Geometry check sheet. Reference: the model listing, model coordinates, mm. A direction names the side the tool comes from. Round coordinates to 2 decimals unless told otherwise and drop trailing zeros. Write each loop counter-clockwise with the first axis right and the second up, starting at its lowest first coordinate (ties: lowest second). Pieces come first, ordered by that corner, then holes. Notation, with made-up numbers: (41.25, 56) - (47.25, 56) arc R18 ccw to (47.25, 71) - close; hole circle Ø5 at (-28, 55.5). An arc over 180 degrees is marked (long way). Return JSON: item names as keys, results as strings.
Autodesk Inventor part; units mm, degrees
ref_plane "Arbeitsebene1" through (0, 0, 7.5) normal (0, 0, 1) x (1, 0, 0)
ref_plane "YZ Plane" through (0, 0, 0) normal (1, 0, 0) x (0, 1, 0)
ref_plane "XZ Plane" through (0, 0, 0) normal (0, 1, 0) x (-1, 0, 0)
sketch "Skizze1" plane through (0, 0, 0) normal (0, 0, 1) x (1, 0, 0)
  line L0 (6.45, 0) -> (15, 0)
  line L1 (15, 0) -> (15, 15)
  line L2 (15, 15) -> (0, 15)
  line L3 (0, 15) -> (0, 3.0582)
  arc A0 (6.45, 0) -> (0, 3.0582) centre (2.5, 0) ccw
  line L4 (-3, 0) -> (18, 0)
  line L5 (0, -3) -> (0, 18)
  point P0 (0, 0)
  dimension "d0" = 15
  dimension "d1" = 15
  dimension "d2" = 7.9
  dimension "d3" = 2.5
extrude "Extrusion1" add sketch "Skizze1" along normal mid plane 17.5 contours A0 L3 L2 L1 L0
ref_plane "Arbeitsebene1" through (0, 0, 7.5) normal (0, 0, 1) x (1, 0, 0)
sketch "Skizze2" plane through (0, 0, 7.5) normal (0, 0, 1) x (1, 0, 0)
  circle A0 centre (2.5, 0) radius 3.95
  arc A1 (6.45, 0) -> (0, 3.0582) centre (2.5, 0) ccw
  circle A2 centre (2.5, 0) radius 3.45
  line L0 (0, 3.0582) -> (0, 2.3775)
  line L1 (15, 0) -> (6.45, 0)
  line L2 (6.45, 0) -> (5.95, 0)
  point P0 (0, 0)
  point P1 (0, 3.0582)
  dimension "d7" = 7.9
  dimension "d8" = 6.9
extrude "Extrusion2" add sketch "Skizze2" against normal up to surface (16.25 mm away) contours L2 A2 L0 A0 picked at (6.25, 0.2945)
sketch "Skizze4" plane through (15, 0, 8.75) normal (1, 0, 0) x (0, 0, -1)
  line L0 (17.5, 3) -> (0, 3)
  line L1 (0, 3) -> (0, 0)
  line L2 (0, 0) -> (17.5, 0)
  line L3 (17.5, 0) -> (17.5, 3)
  line L4 (17.5, 15) -> (17.5, 0)
  line L5 (0, 0) -> (0, 15)
  line L6 (17.5, 0) -> (0, 0)
  point P0 (8.75, 0)
  dimension "d11" = 3
extrude "Extrusion3" add sketch "Skizze4" along normal blind 13
fillet "Rundung1" radius 4 1 edges at (15, 3, 0)
sketch "Skizze5" plane through (28, 3, 8.75) normal (0, 1, 0) x (1, 0, 0)
  line L0 (-9, 0) -> (0, 0)
  line L1 (0, 17.5) -> (0, 0)
  point P0 (-28, 8.75)
  point P1 (-6.5, 10)
  dimension "d15" = 10
  dimension "d16" = 6.5
hole "Bohrung1" at (21.5, 3, -1.25) direction (0, -1, 0) diameter 4.1 end through all
sketch "Skizze6" plane through (5.95, 0, -8.75) normal (0, -1, 0) x (1, 0, 0)
  line L0 (0, 0) -> (22.05, 0)
  line L1 (-11.55, 8.75) -> (27.65, 8.75)
  line L2 (0, 16.25) -> (0, 0)
  point P0 (-5.95, 8.75)
  point P1 (6, 3)
  point P2 (6, 8.75)
  dimension "d24" = 3
  dimension "d25" = 6
hole "Bohrung2" at (11.95, 0, -5.75) at (11.95, 0, 0) direction (0, 1, 0) diameter 4 depth 8 tip angle 118
sketch "Skizze7" plane through (0, 0, -8.75) normal (0, 0, -1) x (-1, 0, 0)
  circle A0 centre (-2.5, 0) radius 6
  arc A1 (0, 2.3775) -> (-5.95, 0) centre (-2.5, 0) ccw
  line L0 (-5.95, 0) -> (-8.5, 0)
  line L1 (-5.95, 0) -> (-28, 0)
  line L2 (0, 2.3775) -> (0, 15)
  line L3 (0, 2.3775) -> (0, 5.4544)
  point P0 (0, 0)
  dimension "d34" = 12
extrude "Extrusion4" cut sketch "Skizze7" against normal blind 14 contours L2 A1 L0 A0 picked at (-7.6008, 0.4409)
chamfer "Fasen1" distance 2 angle 45 1 edges at (3.7801, 3.2037, 5.25)
sketch "Skizze8" plane through (0, 3.0582, 8.75) normal (-1, 0, 0) x (0, 0, 1)
  line L0 (0, 3.9418) -> (0, 11.9418)
  line L1 (0, 3.9418) -> (-0.5, 11.9418)
  line L2 (-17.5, 11.9418) -> (0, 11.9418)
  line L3 (-0.5, 11.9418) -> (0, 11.9418)
  line L4 (0, 11.9418) -> (0, 3.9418)
  point P0 (-8.75, -3.0582)
  dimension "d40" = 8
  dimension "d41" = 0.5
extrude "Extrusion5" cut sketch "Skizze8" against normal through all
equation "\"d0\" = Tiefe_Gegenstueck"
equation "\"d1\" = Breite_Grundkoerper"
equation "\"d2\" = D_Scheibe"
equation "\"d3\" = Abstand_D_Scheibe"
equation "\"d4\" = Tiefe_Grundkoerper"
equation "\"d7\" = D_Scheibe"
equation "\"d11\" = Breite_Absatz"
equation "\"d12\" = Tiefe_Absatz"
equation "\"d14\" = Radius_Absatz"
equation "\"d17\" = D_Kolbenbohrung"
equation "\"d26\" = D_Zentrierbohrung"
equation "\"d31\" = T_Zentrierbohrung"
equation "\"Breite_Grundkoerper\" = 15"
equation "\"D_Scheibe\" = 7.9"
equation "\"Abstand_D_Scheibe\" = 2.5"
equation "\"Abstand_Arbeitsebene\" = 2"
equation "\"Tiefe_Grundkoerper\" = 17.5"
equation "\"Tiefe_Gegenstueck\" = 15"
equation "\"Breite_Absatz\" = 3"
equation "\"Tiefe_Absatz\" = 13"
equation "\"Radius_Absatz\" = 4"
equation "\"Pos_Bohrung_Kolben_x\" = 6.5"
equation "\"Pos_Bohrung_Kolben_y\" = 10"
equation "\"D_Kolbenbohrung\" = 4.1"
equation "\"Zentrierbohrung_y\" = 3"
equation "\"T_Zentrierbohrung\" = 8"
equation "\"D_Zentrierbohrung\" = 4"
equation "\"Zentrierbohrung_x\" = 6"
equation "\"R_Kanten\" = 0.5"
properties part number "JH_int_Greiferkoerper_Gegenstueck"
(1) Section check D-D, the plane y = 4.5. Give the number of separate pieces and of enclosed holes in the cut face, plus the area to 3 significant figures.
Response values:
{"separate pieces": "1", "enclosed holes": "2", "area": "158 mm^2"}
(2) Material ranges on line 1 along Z through (x, y) = (11.95, 4.5); line 2 along X through (y, z) = (2.2, -1.25); line 3 along Y through (x, z) = (23.75, 2.75), recorded low to high. Write a range as [from, to].
Response values:
{"line 1": "z = [-8.75, -7.75], [-3.75, -2], [2, 8.75]", "line 2": "x = [8.08, 10.39], [13.51, 19.45], [23.55, 28]", "line 3": "y = [0, 3]"}
(3) Release check for a two-part mould opening along Z. For faces 1 (the face through (20.884, 1.479, 0.705)), 2 (the face through (14, 4, 8.75)), 3 (the face through (19, 0, 0)), 4 (the face through (13.9, 4.1, -5.3)) record: pulls with the +Z half, pulls with the -Z half, needs draft (parallel to the pull), parting line crosses it, or undercut.
Response values:
{"face 1": "undercut", "face 2": "pulls with the +Z half", "face 3": "needs draft", "face 4": "undercut"}
(4) Section check C-C, the plane z = 5.75. Enter the section's corners in (x, y).
Response values:
{"outline": "(0, 4.27) arc R4.95 cw to (7.45, 0) - (28, 0) - (28, 3) - (19, 3) arc R4 cw to (15, 7) - (15, 15) - (0, 15) - close"}
(5) Section check B-B, the plane y = 11. Enter the section's corners in (x, z).
Response values:
{"outline": "(0, -8.75) - (15, -8.75) - (15, 8.5) - (0, 8.5) - close"}
(6) Section check A-A, the plane x = 21.5. Enter the section's corners in (y, z), plus the area to 3 significant figures.
Response values:
{"outline": "(0, -8.75) - (3, -8.75) - (3, -3.3) - (0, -3.3) - close; (0, 0.8) - (3, 0.8) - (3, 8.75) - (0, 8.75) - close", "area": "40.2 mm^2"}
(7) Gauge pin test, flat ends, axial feed: pin 1 (1 mm diameter, centred on x = 22, z = -3.5, fed in from +Y); pin 2 (6.5 mm diameter, centred on y = 11, z = -2, fed in from +X); pin 3 (3 mm diameter, centred on x = 4.5, y = 2.5, fed in from -Z). Record the tip position at first contact, or that the pin passes through.
Response values:
{"pin 1": "stops at y = 3", "pin 2": "stops at x = 15", "pin 3": "stops at z = 6"}
(8) Access from +Z, -Z, +X, -X, +Y, -Y to the whole of each face (thin tool, end or side, straight path). Record for faces 5 (the face through (0, 10, 0)), 6 (the face through (4.136, 3.595, 8.116)), 7 (the face through (23.4, 3, -0.1)), 8 (the face through (8, 15, 0)), 9 (the face through (5.669, 5.095, -1.848)).
Response values:
{"face 5": "+Z, -Z, -X, +Y, -Y", "face 6": "+Z, -Y", "face 7": "+Z, -Z, +X, +Y", "face 8": "+Z, -Z, +X, -X, +Y", "face 9": "-Z, -Y"}
